```python
from build123d import *

# Parameters (mm, degrees)
SKETCH1_R           = 3
SKETCH1_W           = 130
SKETCH1_H           = 10
BOSS_EXTRUDE1_DEPTH = 10
SKETCH2_W           = 130
SKETCH2_H           = 8.023003322
BOSS_EXTRUDE2_DEPTH = 75
FILLET1_R           = 5
SKETCH3_W           = 130
SKETCH3_H           = 8.023003322
CUT_EXTRUDE1_DEPTH  = 75
SKETCH4_W           = 130
SKETCH4_H           = 10
CUT_EXTRUDE2_DEPTH  = 37
SKETCH5_W           = 130
SKETCH5_H           = 10
BOSS_EXTRUDE4_DEPTH = 75
FILLET2_R           = 5
SKETCH6_R           = 10
SKETCH6_R_2         = 7.5
SKETCH6_R_3         = 3.5
SKETCH6_R_4         = 2.5
CUT_EXTRUDE3_DEPTH  = 10
SKETCH7_R           = 19.1
CUT_EXTRUDE4_DEPTH  = 10
SKETCH8_R           = 3.5
BOSS_EXTRUDE5_DEPTH = 10


with BuildPart() as part:
    # Sketch1 → Boss-Extrude1 (new body)
    # profile 1 of 3: a face of its own
    with BuildSketch(Plane(origin=(0, 0, 0), x_dir=(1, 0, 0), z_dir=(0, 1, 0))):
        Polygon((0, 63), (0, 0), (5, 0), (130, 0), (130, 63), align=None)
        with Locations(Location((5, 17, 0), (0, 0, 270))):
            Circle(SKETCH1_R, mode=Mode.SUBTRACT)
        with Locations(Location((45, 17, 0), (0, 0, 270))):
            Circle(SKETCH1_R, mode=Mode.SUBTRACT)
        with Locations(Location((5, 57, 0), (0, 0, 270))):
            Circle(SKETCH1_R, mode=Mode.SUBTRACT)
        with Locations(Location((45, 57, 0), (0, 0, 270))):
            Circle(SKETCH1_R, mode=Mode.SUBTRACT)
        with Locations(Location((85, 17, 0), (0, 0, 270))):
            Circle(SKETCH1_R, mode=Mode.SUBTRACT)
        with Locations(Location((125, 17, 0), (0, 0, 270))):
            Circle(SKETCH1_R, mode=Mode.SUBTRACT)
        with Locations(Location((85, 57, 0), (0, 0, 270))):
            Circle(SKETCH1_R, mode=Mode.SUBTRACT)
        with Locations(Location((125, 57, 0), (0, 0, 270))):
            Circle(SKETCH1_R, mode=Mode.SUBTRACT)
    # profile 2 of 3: a face of its own
    with BuildSketch(Plane(origin=(0, 0, 0), x_dir=(1, 0, 0), z_dir=(0, 1, 0))):
        Polygon((5, 0), (0, 0), (0, -27), (130, -27), (130, 0), align=None)
    # profile 3 of 3: a face of its own
    with BuildSketch(Plane(origin=(0, 0, 0), x_dir=(1, 0, 0), z_dir=(0, 1, 0))):
        with Locations((65, -32)):
            Rectangle(SKETCH1_W, SKETCH1_H)
    extrude(amount=BOSS_EXTRUDE1_DEPTH)

    # Sketch2 → Boss-Extrude2 (add)
    with BuildSketch(Plane(origin=(0, 10, 0), x_dir=(1, 0, 0), z_dir=(0, 1, 0))):
        with Locations((65, -32.988498339)):
            Rectangle(SKETCH2_W, SKETCH2_H)
    extrude(amount=BOSS_EXTRUDE2_DEPTH)

    # Fillet1
    fillet1_edges = [part.edges().sort_by_distance(p)[0] for p in [
        (0, 85, 32.988498339),
        (130, 85, 32.988498339),
        (130, 5, -63),
        (0, 5, -63),
    ]]
    fillet(fillet1_edges, radius=FILLET1_R)

    # Sketch3 → Cut-Extrude1 (cut)
    with BuildSketch(Plane(origin=(0, 85, 0), x_dir=(1, 0, 0), z_dir=(0, 1, 0))):
        with Locations((65, -32.988498339)):
            Rectangle(SKETCH3_W, SKETCH3_H)
    extrude(amount=-CUT_EXTRUDE1_DEPTH, mode=Mode.SUBTRACT)

    # Sketch4 → Cut-Extrude2 (cut)
    with BuildSketch(Plane.XY.offset(37)):
        with Locations((65, 5)):
            Rectangle(SKETCH4_W, SKETCH4_H)
    extrude(amount=-CUT_EXTRUDE2_DEPTH, mode=Mode.SUBTRACT)

    # Sketch5 → Boss-Extrude4 (add)
    with BuildSketch(Plane(origin=(0, 10, 0), x_dir=(1, 0, 0), z_dir=(0, 1, 0))):
        with Locations((65, 5)):
            Rectangle(SKETCH5_W, SKETCH5_H)
    extrude(amount=BOSS_EXTRUDE4_DEPTH)

    # Fillet2
    fillet2_edges = [part.edges().sort_by_distance(p)[0] for p in [
        (130, 85, -5),
        (0, 85, -5),
    ]]
    fillet(fillet2_edges, radius=FILLET2_R)

    # Sketch6 → Cut-Extrude3 (cut)
    with BuildSketch(Plane(origin=(0, 0, -10), x_dir=(-1, 0, 0), z_dir=(0, 0, -1))):
        with Locations((-113, 47.5)):
            Circle(SKETCH6_R)
        with Locations((-65, 47.5)):
            Circle(SKETCH6_R_2)
        with Locations((-17, 47.5)):
            Circle(SKETCH6_R)
        with Locations((-113, 71.5)):
            Circle(SKETCH6_R_3)
        with Locations((-65, 74.04)):
            Circle(SKETCH6_R_3)
        with Locations((-17, 71.5)):
            Circle(SKETCH6_R_3)
        with Locations((-17, 23.5)):
            Circle(SKETCH6_R_3)
        with Locations((-65, 21)):
            Circle(SKETCH6_R_3)
        with Locations((-113, 23.5)):
            Circle(SKETCH6_R_3)
        with Locations((-88.58, 71.06)):
            Circle(SKETCH6_R_4)
        with Locations((-41.44, 71.06)):
            Circle(SKETCH6_R_4)
        with Locations((-41.44, 23.92)):
            Circle(SKETCH6_R_4)
        with Locations((-88.58, 23.92)):
            Circle(SKETCH6_R_4)
    extrude(amount=-CUT_EXTRUDE3_DEPTH, mode=Mode.SUBTRACT)

    # Sketch7 → Cut-Extrude4 (cut)
    with BuildSketch(Plane(origin=(0, 0, -10), x_dir=(-1, 0, 0), z_dir=(0, 0, -1))):
        with Locations((-65, 47.5)):
            Circle(SKETCH7_R)
    extrude(amount=-CUT_EXTRUDE4_DEPTH, mode=Mode.SUBTRACT)

    # Sketch8 → Boss-Extrude5 (add)
    with BuildSketch(Plane(origin=(0, 0, -10), x_dir=(-1, 0, 0), z_dir=(0, 0, -1))):
        with Locations((-65, 74.04)):
            Circle(SKETCH8_R)
        with Locations((-65, 21)):
            Circle(SKETCH8_R)
    extrude(amount=-BOSS_EXTRUDE5_DEPTH)


solid = part.part
```
The model under review builds one solid part; all positions refer to its coordinate system, in mm. A direction names the side the tool comes from. Give positions to 0.01 mm unless a question says otherwise; leave off trailing zeros. Write each loop counter-clockwise with the first axis right and the second up, starting at its lowest first coordinate (ties: lowest second). Pieces come first, ordered by that corner, then holes.
(1) Consider section D-D, the plane y = 31.5. Give the boundary of the cut face in (x, z), and give its area (3 significant figures).
(2) Tool access review of faces 1 (the cylindrical face through (83.2, 4.9, -59.4)), 2 (the flat face through (64, 10, -37)): name each direction out of +Z, -Z, +X, -X, +Y, -Y from which nothing blocks a thin tool from reaching the whole face with its end or side.
(3) Consider section A-A, the plane x = 113. Give the boundary of the cut face in (y, z).
(4) Consider section B-B, the plane y = 55. Give the boundary of the cut face in (x, z), and give its area (3 significant figures).
(5) To check wall thickness, follow L1, parallel to Y at x = 88.58, z = -4.5; L2, parallel to X at y = 23, z = -7; L3, parallel to X at y = 53.5, z = -6.5. State the ranges of each line that lie inside material, in increasing order.
(6) For P1, Ø5, axis at x = 84.5, z = -18, coming from the +Y side; P2, Ø4, axis at x = 17, y = 23.5, coming from the +Z side; P3, Ø8, axis at x = 100.5, y = 34, coming from the -Z side, all flat-tipped, find the tip position at first contact; note any pin that passes through.
(7) The part is to be moulded in two halves that separate along X. For faces 3 (the flat face through (64, 85, -5)), 4 (the cylindrical face through (41.77, 73.54, -5.07)), 5 (the flat face through (130, 28, -9.5)), 6 (the cylindrical face through (115.17, 37.74, -5.07)), say which applies: released by +X, released by -X, zero draft, split by the parting line, or undercut.
(8) Consider section C-C, the plane x = 80.5. Give the boundary of the cut face in (y, z), and give its area (3 significant figures).
Returned:
1. outline: (0, -10) - (54.57, -10) - (54.57, 0) - (0, 0) - close; (75.43, -10) - (130, -10) - (130, 0) - (75.43, 0) - close
1. area: 1,090 mm2
2. face 1: +Y, -Y
2. face 2: -Z, +X, -X, +Y
3. outline: (0, -63) - (10, -63) - (10, -10) - (20, -10) - (20, 0) - (0, 0) - close; (27, -10) - (37.5, -10) - (37.5, 0) - (27, 0) - close; (57.5, -10) - (68, -10) - (68, 0) - (57.5, 0) - close; (75, -10) - (85, -10) - (85, 0) - (75, 0) - close
4. outline: (0, -10) - (10.39, -10) - (10.39, 0) - (0, 0) - close; (23.61, -10) - (47.43, -10) - (47.43, 0) - (23.61, 0) - close; (82.57, -10) - (106.39, -10) - (106.39, 0) - (82.57, 0) - close; (119.61, -10) - (130, -10) - (130, 0) - (119.61, 0) - close
4. area: 684 mm2
5. L1: y = 0 to 21.42, 26.42 to 68.56, 73.56 to 85
5. L2: x = 0 to 13.54, 20.46 to 39.12, 43.76 to 86.26, 90.9 to 109.54, 116.46 to 130
5. L3: x = 0 to 9, 25 to 46.87, 83.13 to 105, 121 to 130
6. P1: stops at y = 10
6. P2: passes through
6. P3: stops at z = -10
7. face 3: zero draft
7. face 4: undercut
7. face 5: released by +X
7. face 6: undercut
8. outline: (0, -63) - (10, -63) - (10, -10) - (36.34, -10) - (36.34, 0) - (0, 0) - close; (58.66, -10) - (85, -10) - (85, 0) - (58.66, 0) - close
8. area: 1,160 mm2
